Read the model definition and answer for the solid it produces. Units are mm, in the model's axes. A direction names the side the tool comes from. Coordinates: 2 decimals unless noted, no trailing zeros. Write each loop counter-clockwise with the first axis right and the second up, starting at its lowest first coordinate (ties: lowest second). Pieces come first, ordered by that corner, then holes. Notation, with made-up numbers: (-12, 26) -> (-8, 26) arc R18 cw to (-8, 55) -> close; hole circle Ø9 at (-1.5, 22.25). An arc over 180 degrees is marked (long way). Answer as a JSON object with one key per item and string values. Group by question number.
(1) Flat-ended cylindrical pins translate along their axes: P1, Ø4, axis at y = 109, z = 158.5, coming from the -X side; P2, Ø2, axis at y = 173, z = 145.5, coming from the +X side; P3, Ø3, axis at x = 22.5, z = 299.5, coming from the -Y side. Find the tip coordinate at first contact, or state that the pin passes through.
(2) Find section B-B (x = 148). Give the vertices of the cut face in (y, z), then the cut area to 3 significant figures.
(3) Which of the six approach directions +Z, -Z, +X, -X, +Y, -Y give full straight-line access (tool end or side, diameter ignored) to faces 1 (the face through (-42.897, 201, 214)), 2 (the face through (158, 1, 214))?
(4) Find section C-C (y = 174.5). Give the vertices of the cut face in (x, z), then the cut area to 3 significant figures.
(5) Find section A-A (z = 397). Give the vertices of the cut face in (x, y).
(6) Straight lines are drawn through the part: L1, parallel to Y at x = 167, z = 313; L2, parallel to X at y = 167.5, z = 137; L3, parallel to Y at x = 75, z = 31.5. For each, find the intervals that lie inside material, in ascending order.
from build123d import *

# Parameters (mm, degrees)
BOSS_EXTRUDE1_DEPTH = 490
SKETCH3_W           = 307.381871045
SKETCH3_H           = 276.781214979
CUT_EXTRUDE1_DEPTH  = 55


with BuildPart() as part:
    # Sketch1 → Boss-Extrude1 (new body)
    with BuildSketch(Plane.XY):
        with BuildLine():
            Line((-42.896935933, 250), (-42.896935933, 150))
            ThreePointArc((-42.896935933, 150), (1.037046889, 43.933982822), (107.103064067, 0))
            Line((107.103064067, 0), (207.103064067, 0))
            Line((207.103064067, 0), (207.103064067, 1))
            Line((207.103064067, 1), (107.103064067, 1))
            ThreePointArc((107.103064067, 1), (1.74415367, 44.641089603), (-41.896935933, 150))
            Line((-41.896935933, 150), (-41.896935933, 250))
            Line((-41.896935933, 250), (-42.896935933, 250))
        make_face()
    extrude(amount=BOSS_EXTRUDE1_DEPTH)

    # Sketch3 → Cut-Extrude1 (cut)
    with BuildSketch(Plane.XY.offset(490)):
        with Locations((90.01109878, 115.028999709)):
            Rectangle(SKETCH3_W, SKETCH3_H)
    extrude(amount=-CUT_EXTRUDE1_DEPTH, mode=Mode.SUBTRACT)


solid = part.part
Results below:
{
 "1": {"P1": "stops at x = -37.74", "P2": "stops at x = -41.9", "P3": "stops at y = 25.12"},
 "2": {"outline": "(0, 0) -> (1, 0) -> (1, 435) -> (0, 435) -> close", "area": "435 mm2"},
 "3": {"face 1": "+Z, -Z, -X, +Y, -Y", "face 2": "+Z, -Z, +X, +Y"},
 "4": {"outline": "(-42.9, 0) -> (-41.9, 0) -> (-41.9, 435) -> (-42.9, 435) -> close", "area": "435 mm2"},
 "5": {"outline": "(-42.9, 150) arc R150 ccw to (107.1, 0) -> (207.1, 0) -> (207.1, 1) -> (107.1, 1) arc R149 cw to (-41.9, 150) -> (-41.9, 250) -> (-42.9, 250) -> close"},
 "6": {"L1": "y = 0 to 1", "L2": "x = -42.9 to -41.9", "L3": "y = 3.48 to 4.5"}
}
